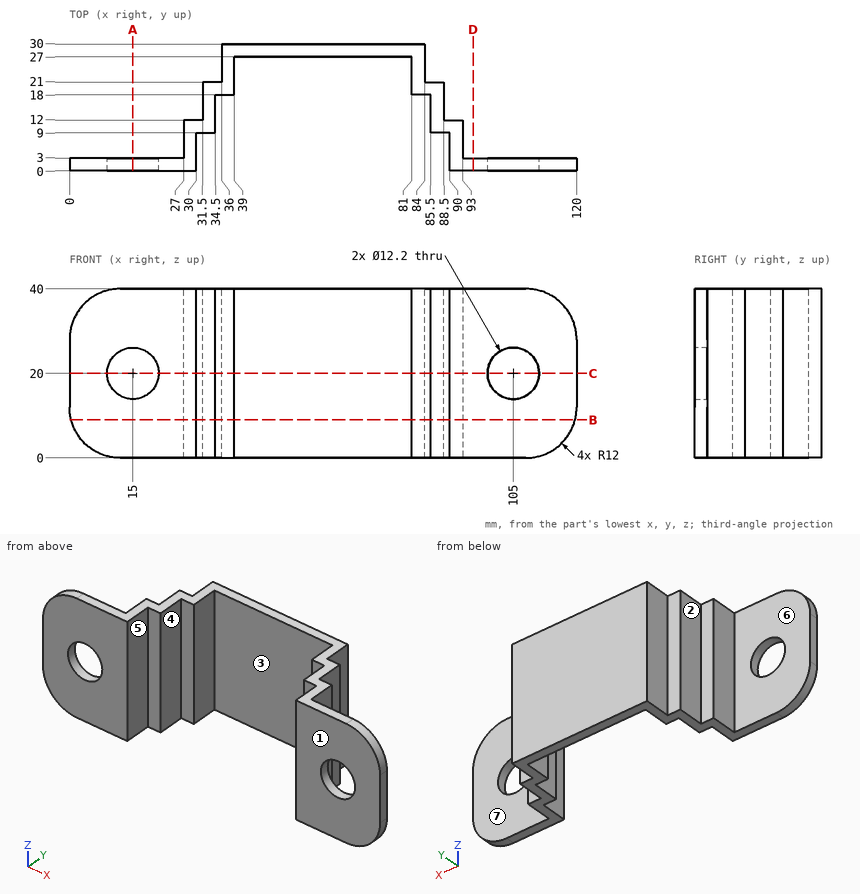
Geometry: see drawing. Coordinates: mm, zero at the bounding-box minimum. A direction names the side the tool comes from. Give positions to 0.01 mm unless a question says otherwise; leave off trailing zeros. Loops run counter-clockwise (first coordinate to the right, second up) from the corner with the lowest first, then second, coordinate; pieces in that order, holes last. Notation, with made-up numbers: M 88.5,41.25 L 106.5,41.25 A9 ccw 106.5,51.25 Z; hole C 10.5,8.5 d11. An arc over 180 degrees is marked long. Answer as CSV lines item,"result". Start each with the question number.
1. Section B-B on z = 9. Return loops of the section in (x, y).
2. Section C-C on z = 20. State how many separate pieces and enclosed holes the cut face has, plus the area to 3 significant figures.
3. Reachability of the marked faces 5, 6 and 7 from +Z, -Z, +X, -X, +Y, -Y: full face, straight path, thin tool, end or side. Return the list, or none.
4. Section A-A on x = 15. Return loops of the section in (y, z).
5. Section D-D on x = 95.5. Return loops of the section in (y, z), plus the area to 3 significant figures.
6. Pull-direction query (X, two-part tool) for the marked faces 1, 2, 3 and 4; classes: released by +X, released by -X, zero draft, split by the parting line, or undercut.
7. Line query: L1, parallel to X at y = 1.75, z = 20; L2, parallel to X at y = 12.75, z = 25; L3, parallel to X at y = 8, z = 25.5. Output: solid intervals per line, ascending.
8. Pin query (flat end, axial travel): P1, Ø2.5, axis at y = 25, z = 14.5, coming from the +X side; P2, Ø2.5, axis at y = 13, z = 27, coming from the -X side; P3, Ø7, axis at y = 15, z = 15.5, coming from the +X side. Return the tip coordinate at first contact, or that it passes through.
Computed values:
1,outline,"M 0.38,0 L 30,0 L 30,9 L 34.5,9 L 34.5,18 L 39,18 L 39,27 L 81,27 L 81,18 L 85.5,18 L 85.5,9 L 90,9 L 90,0 L 119.62,0 L 119.62,3 L 93,3 L 93,12 L 88.5,12 L 88.5,21 L 84,21 L 84,30 L 36,30 L 36,21 L 31.5,21 L 31.5,12 L 27,12 L 27,3 L 0.38,3 Z"
2,separate pieces,"3"
2,enclosed holes,"0"
2,area,"449 mm²"
3,face 5,"+Z, -Z, -Y"
3,face 6,"+Z, -Z, -X, +Y"
3,face 7,"+Z, -Z, +X, +Y"
4,outline,"M 0,0 L 3,0 L 3,13.9 L 0,13.9 Z; M 0,26.1 L 3,26.1 L 3,40 L 0,40 Z"
5,outline,"M 0,0 L 3,0 L 3,40 L 0,40 Z"
5,area,"120 mm²"
6,face 1,"zero draft"
6,face 2,"released by -X"
6,face 3,"undercut"
6,face 4,"undercut"
7,L1,"x = 0 to 8.9, 21.1 to 30, 90 to 98.9, 111.1 to 120"
7,L2,"x = 31.5 to 34.5, 85.5 to 88.5"
7,L3,"x = 27 to 30, 90 to 93"
8,P1,"stops at x = 84"
8,P2,"stops at x = 27"
8,P3,"stops at x = 93"
